Work out the finished part from the listing and answer in its coordinate system (mm). A direction names the side the tool comes from. Coordinates: 2 decimals unless noted, no trailing zeros. Loops run counter-clockwise (first coordinate to the right, second up) from the corner with the lowest first, then second, coordinate; pieces in that order, holes last. Notation, with made-up numbers: (28.5, 27.25) - (67.5, 27.25) arc R17 ccw to (67.5, 53.25) - close; hole circle Ø11 at (69, 86). An arc over 180 degrees is marked (long way). Write each question's results on one line, items separated by ' | '. Start each with the question number.
1. Which of the six approach directions +Z, -Z, +X, -X, +Y, -Y give full straight-line access (tool end or side, diameter ignored) to faces 4 (the flat face through (0, 0, 62)), 5 (the cylindrical face through (14, -15.43, 35.78))?
2. Determine the mould class of faces 1 (the flat face through (15, 16, 33.5)), 2 (the flat face through (-21, 0, 19)), 3 (the flat face through (18.3, -18.2, 18.7)) for opening direction Y: released by +Y, released by -Y, zero draft, split by the parting line, or undercut.
3. A cutting plane is placed at B-B on y = 0. Determine the outline of the cut face in (x, z), then the cut area to 3 significant figures.
4. Find the intervals of material crossed by line 1 along Y through (x, z) = (-15.5, 37); line 2 along Z through (x, y) = (-10.5, 19); line 3 along Y through (x, z) = (-15, 35), in increasing order. Write a range as [from, to].
5. Each of these flat-tipped pins is pushed along its axis until it touches: P1, Ø2.5, axis at x = 15.5, y = -15.5, coming from the +Z side; P2, Ø8, axis at x = 9.5, y = 15, coming from the +Z side. Where does it stop, or does it pass through?
6. A cutting plane is placed at A-A on z = 9.5. Determine the outline of the cut face in (x, y), then the cut area to 3 significant figures.
7. A cutting plane is placed at D-D on y = -7.5. Determine the outline of the cut face in (x, z).
from build123d import *

# Parameters (mm, degrees)
PAD_DEPTH    = 38
SKETCH001_R  = 1.5
POCKET_DEPTH = 4.5
SKETCH002_R  = 11
PAD001_DEPTH = 2
SKETCH003_R  = 2.5
PAD002_DEPTH = 22


with BuildPart() as part:
    # Sketch → Pad (new body)
    with BuildSketch(Plane.XY):
        Polygon((-21, 15.5), (-15.5, 21), (15.5, 21), (21, 15.5), (21, -15.5), (15.5, -21), (-15.5, -21), (-21, -15.5), align=None)
    extrude(amount=PAD_DEPTH)

    # Sketch001 (on Face10 of Pad) → Pocket (cut)
    with BuildSketch(Plane.XY.offset(38)):
        with Locations((-15.5, 15.5)):
            Circle(SKETCH001_R)
        with Locations((15.5, 15.5)):
            Circle(SKETCH001_R)
        with Locations((15.5, -15.5)):
            Circle(SKETCH001_R)
        with Locations((-15.5, -15.5)):
            Circle(SKETCH001_R)
    extrude(amount=-POCKET_DEPTH, mode=Mode.SUBTRACT)

    # Sketch002 (on Face5 of Pocket) → Pad001 (join)
    with BuildSketch(Plane.XY.offset(38)):
        Circle(SKETCH002_R)
    extrude(amount=PAD001_DEPTH)

    # Sketch003 (on Face17 of Pad001) → Pad002 (join)
    with BuildSketch(Plane.XY.offset(40)):
        Circle(SKETCH003_R)
    extrude(amount=PAD002_DEPTH)


solid = part.part
Values:
1) face 4: +Z, +X, -X, +Y, -Y | face 5: +Z
2) face 1: undercut | face 2: zero draft | face 3: released by -Y
3) outline: (-21, 0) - (21, 0) - (21, 38) - (11, 38) - (11, 40) - (2.5, 40) - (2.5, 62) - (-2.5, 62) - (-2.5, 40) - (-11, 40) - (-11, 38) - (-21, 38) - close | area: 1,750 mm^2
4) line 1: [-21, -17], [-14, 14], [17, 21] | line 2: [0, 38] | line 3: [-21, -16.91], [-14.09, 14.09], [16.91, 21]
5) P1: z = 33.5 | P2: z = 38
6) outline: (-21, -15.5) - (-15.5, -21) - (15.5, -21) - (21, -15.5) - (21, 15.5) - (15.5, 21) - (-15.5, 21) - (-21, 15.5) - close | area: 1,700 mm^2
7) outline: (-21, 0) - (21, 0) - (21, 38) - (8.05, 38) - (8.05, 40) - (-8.05, 40) - (-8.05, 38) - (-21, 38) - close
